Job drawing, mm, ordinate dimensions from the low corner. One solid piece. A direction names the side the tool comes from. Round coordinates to 2 decimals unless told otherwise and drop trailing zeros. Order: outer loops, then holes, each group sorted by start corner. A loop starts at its lowest first (then second) coordinate and runs counter-clockwise, first axis right, second up. Notation, with made-up numbers: (42.5, 33) -> (87.5, 33) arc R12 cw to (87.5, 51) -> close; hole circle Ø4 at (-26, -4). An arc over 180 degrees is marked (long way). Answer as a JSON object with one key per item and string values. Group by question number.
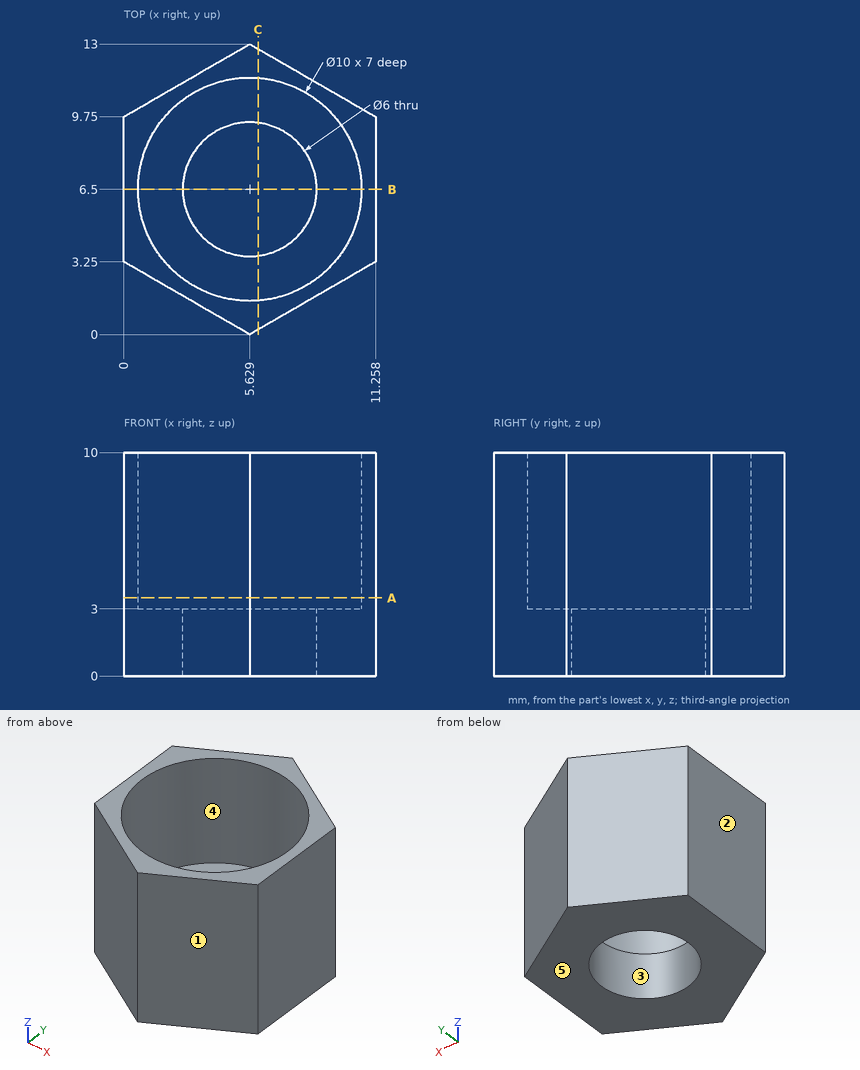
Q1. Drop flat-ended pins along their axis: pin 1 Ø3 at (x, y) = (2.5, 6.5) entering from +Z; pin 2 Ø5 at (x, y) = (8, 4) entering from -Z; pin 3 Ø2 at (x, z) = (2.5, 2) entering from +Y; pin 4 Ø6 at (x, z) = (6, 7) entering from +Y. Give the stop position or say it passes through.
Q2. Two-plate mould, pull along Y, no slides. Class the marked faces 1, 2 and 3: +Y half, -Y half, draft (parallel to the pull), parting line (faces both ways), or undercut.
Q3. Band-saw the part on A-A (z = 3.5). List the corners of the cut face in (x, y).
Q4. Wall check: line 1 (X direction, y = 6.5, z = 2.4); line 2 (X direction, y = 6.5, z = 5); line 3 (Z direction, x = 8.75, y = 8). Give the ranges that are in metal, low to high. Write a range as [from, to].
Q5. Which spindle directions (+Z, -Z, +X, -X, +Y, -Y) get a long thin tool onto all of the face, cutting with end or side? Do the marked faces 4 and 5. Say none if no direction does.
Q6. Band-saw the part on C-C (x = 6). List the corners of the cut face in (y, z).
Q7. Band-saw the part on B-B (y = 6.5). List the corners of the cut face in (x, z).
Completed:
{
 "1": {"pin 1": "z = 3", "pin 2": "z = 0", "pin 3": "y = 11.77", "pin 4": "y = 13"},
 "2": {"face 1": "-Y half", "face 2": "draft", "face 3": "undercut"},
 "3": {"outline": "(0, 3.25) -> (5.63, 0) -> (11.26, 3.25) -> (11.26, 9.75) -> (5.63, 13) -> (0, 9.75) -> close; hole circle Ø10 at (5.63, 6.5)"},
 "4": {"line 1": "[0, 2.63], [8.63, 11.26]", "line 2": "[0, 0.63], [10.63, 11.26]", "line 3": "[0, 3]"},
 "5": {"face 4": "+Z", "face 5": "-Z, +X, -X, +Y, -Y"},
 "6": {"outline": "(0.21, 0) -> (3.52, 0) -> (3.52, 3) -> (1.51, 3) -> (1.51, 10) -> (0.21, 10) -> close; (9.48, 0) -> (12.79, 0) -> (12.79, 10) -> (11.49, 10) -> (11.49, 3) -> (9.48, 3) -> close"},
 "7": {"outline": "(0, 0) -> (2.63, 0) -> (2.63, 3) -> (0.63, 3) -> (0.63, 10) -> (0, 10) -> close; (8.63, 0) -> (11.26, 0) -> (11.26, 10) -> (10.63, 10) -> (10.63, 3) -> (8.63, 3) -> close"}
}
